The model under review builds one solid part; all positions refer to its coordinate system, in mm. Face numbers are marked on the shaded views. A direction names the side the tool comes from. Coordinates: 2 decimals unless noted, no trailing zeros. Loops run counter-clockwise (first coordinate to the right, second up) from the corner with the lowest first, then second, coordinate; pieces in that order, holes last. Notation, with made-up numbers: (56, -29) - (65, -29) arc R29 ccw to (65, 10) - close; hole circle Ø7 at (19, -30.75). An arc over 180 degrees is marked (long way). Answer in a Markdown table with one row per item. Add a question column.
(1) For P1, Ø4, axis at x = 2, y = 10.5, coming from the -Z side; P2, Ø3.5, axis at x = -30.48, z = -11.34, coming from the -Y side, all flat-tipped, find the tip position at first contact; note any pin that passes through.
(2) Mouldability with a two-part tool opening along X and no side actions: class the marked faces 3, 4, 5 and 6 as +X half, -X half, draft (parallel to the pull), parting line (faces both ways), or undercut.
(3) We need section B-B on x = -30.48. Write out the cut boundary in (y, z), plus the area to 3 significant figures.
(4) We need section C-C on y = 16.75. Write out the cut boundary in (x, z) (3 decimals).
(5) We need section D-D on y = 1.75. Write out the cut boundary in (x, z) (3 decimals), plus the area to 3 significant figures.
(6) Machinability: for the marked faces 1 and 2, which of the approach directions +Z, -Z, +X, -X, +Y, -Y give a long, thin tool a straight path to every point of the face, cutting with its end or side? Answer none if there is none.
(7) We need section A-A on z = -0.5. Write out the cut boundary in (x, y) (3 decimals).
(8) For line 1 along X through (y, z) = (14.5, 9.5) (3 decimals); line 2 along Z through (x, y) = (17.5, 19.5); line 3 along X through (y, z) = (4, -11) (3 decimals), list the stretches that pass through material, from the lowest coordinate up.
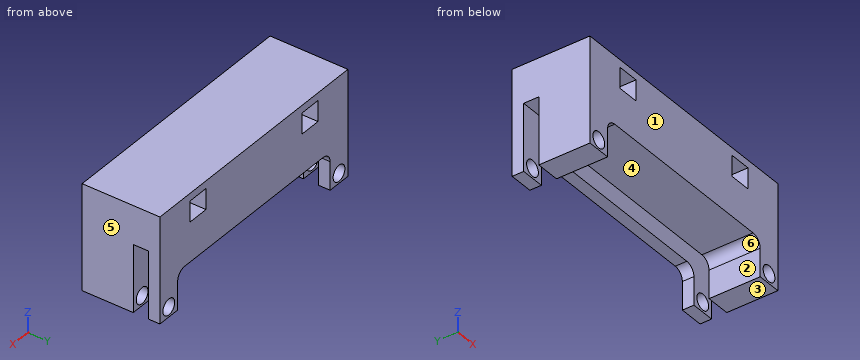
from build123d import *

# Parameters (mm, degrees)
BOSS_EXTRUDE1_DEPTH     = 20.574
CUT_EXTRUDE1_DEPTH      = 3.81
CUT_EXTRUDE1_DEPTH_BACK = 14.224
SKETCH3_W               = 67.31
SKETCH3_H               = 4
SKETCH4_R               = 2.105577283
CUT_EXTRUDE2_DEPTH      = 42.846259104
SKETCH6_W               = 5.8
SKETCH6_H               = 5.5
CUT_EXTRUDE3_DEPTH      = 42.846259104


with BuildPart() as part:
    # Sketch2 → Boss-Extrude1 (new body)
    with BuildSketch(Plane(origin=(0, 0, 0), x_dir=(1, 0, 0), z_dir=(0, 1, 0))):
        with BuildLine():
            Line((-33.655, 13.97), (-27.305, 13.97))
            Line((-27.305, 13.97), (-27.305, 6.51))
            ThreePointArc((-27.305, 6.51), (-26.561051224, 4.713948776), (-24.765, 3.97))
            Line((-24.765, 3.97), (24.765, 3.97))
            ThreePointArc((24.765, 3.97), (26.561051224, 4.713948776), (27.305, 6.51))
            Line((27.305, 6.51), (27.305, 13.97))
            Line((27.305, 13.97), (33.655, 13.97))
            Line((33.655, 13.97), (33.655, -13.97))
            Line((33.655, -13.97), (-33.655, -13.97))
            Line((-33.655, -13.97), (-33.655, 13.97))
        make_face()
    extrude(amount=BOSS_EXTRUDE1_DEPTH)

    # Sketch3 → Cut-Extrude1 (cut, two sides: drawn at the far end of the back side and taken through both)
    with BuildSketch(Plane.XY.offset(-CUT_EXTRUDE1_DEPTH_BACK)):
        with Locations((0, 15.526)):
            Rectangle(SKETCH3_W, SKETCH3_H)
    extrude(amount=CUT_EXTRUDE1_DEPTH + CUT_EXTRUDE1_DEPTH_BACK, mode=Mode.SUBTRACT)

    # Sketch4 → Cut-Extrude2 (cut, through all)
    with BuildSketch(Plane(origin=(0, 20.574, 0), x_dir=(1, 0, 0), z_dir=(0, 1, 0))):
        with Locations(Location((-30.48, 11.337723829, 0), (0, 0, 270))):
            Circle(SKETCH4_R)
        with Locations(Location((30.48, 11.337723829, 0), (0, 0, 90))):
            Circle(SKETCH4_R)
    extrude(amount=-CUT_EXTRUDE2_DEPTH, mode=Mode.SUBTRACT)

    # Sketch6 → Cut-Extrude3 (cut, through all)
    with BuildSketch(Plane(origin=(0, 20.574, 0), x_dir=(1, 0, 0), z_dir=(0, 1, 0))):
        with Locations((20.045, -9.22)):
            Rectangle(SKETCH6_W, SKETCH6_H)
        with Locations((-20.045, -9.22)):
            Rectangle(SKETCH6_W, SKETCH6_H)
    extrude(amount=-CUT_EXTRUDE3_DEPTH, mode=Mode.SUBTRACT)


solid = part.part
Outcome:
| question | item | result |
|---|---|---|
| 1 | P1 | z = -3.97 |
| 1 | P2 | through |
| 2 | face 3 | draft |
| 2 | face 4 | undercut |
| 2 | face 5 | +X half |
| 2 | face 6 | undercut |
| 3 | outline | (0, -13.97) - (13.53, -13.97) - (13.53, -13.44) - (0, -13.44) - close; (0, -9.23) - (13.53, -9.23) - (13.53, 3.81) - (17.53, 3.81) - (17.53, -9.23) - (20.57, -9.23) - (20.57, 13.97) - (0, 13.97) - close; (17.53, -13.97) - (20.57, -13.97) - (20.57, -13.44) - (17.53, -13.44) - close |
| 3 | area | 434 mm² |
| 4 | outline | (-33.655, 3.81) - (33.655, 3.81) - (33.655, 13.97) - (-33.655, 13.97) - close; hole (-22.945, 6.47) - (-17.145, 6.47) - (-17.145, 11.97) - (-22.945, 11.97) - close; hole (17.145, 6.47) - (22.945, 6.47) - (22.945, 11.97) - (17.145, 11.97) - close |
| 5 | outline | (-33.655, -13.97) - (-27.305, -13.97) - (-27.305, -6.51) arc R2.54 cw to (-24.765, -3.97) - (24.765, -3.97) arc R2.54 cw to (27.305, -6.51) - (27.305, -13.97) - (33.655, -13.97) - (33.655, 13.97) - (-33.655, 13.97) - close; hole circle Ø4.211 at (-30.48, -11.338); hole (-22.945, 6.47) - (-17.145, 6.47) - (-17.145, 11.97) - (-22.945, 11.97) - close; hole (17.145, 6.47) - (22.945, 6.47) - (22.945, 11.97) - (17.145, 11.97) - close; hole circle Ø4.211 at (30.48, -11.338) |
| 5 | area | 1,250 mm² |
| 6 | face 1 | +Z, -Z, +X, -X, -Y |
| 6 | face 2 | -Z, +Y, -Y |
| 7 | outline | (-33.655, 0) - (33.655, 0) - (33.655, 13.526) - (-33.655, 13.526) - close; (-33.655, 17.526) - (33.655, 17.526) - (33.655, 20.574) - (-33.655, 20.574) - close |
| 8 | line 1 | -33.655 to -22.945, -17.145 to 17.145, 22.945 to 33.655 |
| 8 | line 2 | -3.97 to 6.47, 11.97 to 13.97 |
| 8 | line 3 | -33.655 to -32.558, -28.402 to -27.305, 27.305 to 28.402, 32.558 to 33.655 |
